Source: CAD feature listing. Evaluate the final solid. Frame: model axes, mm. A direction names the side the tool comes from. Coordinates: 2 decimals unless noted, no trailing zeros. Loops run counter-clockwise (first coordinate to the right, second up) from the corner with the lowest first, then second, coordinate; pieces in that order, holes last.
Autodesk Inventor part; units mm, degrees
ref_plane "YZ Plane" through (0, 0, 0) normal (1, 0, 0) x (0, 1, 0)
ref_plane "XZ Plane" through (0, 0, 0) normal (0, 1, 0) x (-1, 0, 0)
ref_plane "XY Plane" through (0, 0, 0) normal (0, 0, 1) x (1, 0, 0)
sketch "Boceto1" plane through (0, 0, 0) normal (0, 1, 0) x (-1, 0, 0)
  line L0 (-25, 24.85) -> (25, 24.85)
  line L1 (25, 24.85) -> (25, -24.85)
  line L2 (25, -24.85) -> (-25, -24.85)
  line L3 (-25, -24.85) -> (-25, 24.85)
  line L4 (-25, 24.85) -> (25, -24.85) construction
  line L5 (25, 24.85) -> (-25, -24.85) construction
  circle A0 centre (0, 0) radius 4.35
  dimension "d0" = 50
  dimension "d1" = 8.7
  dimension "d2" = 49.7
extrude "Extrusión1" add sketch "Boceto1" along normal blind 10
sketch "Boceto4" plane through (0, 0, 0) normal (0, -1, 0) x (1, 0, 0)
  line L0 (25, 24.85) -> (25, -24.85)
  line L1 (-25, -24.85) -> (-25, 24.85)
  line L2 (25, 24.85) -> (-25, 24.85)
  line L3 (-25, 24.85) -> (-25, 17.85)
  line L4 (-25, 17.85) -> (25, 17.85)
  line L5 (25, 17.85) -> (25, 24.85)
  line L6 (25, -24.85) -> (-25, -24.85)
  line L7 (25, -24.85) -> (-25, -24.85)
  line L8 (-25, -24.85) -> (-25, -17.85)
  line L9 (-25, -17.85) -> (25, -17.85)
  line L10 (25, -17.85) -> (25, -24.85)
  line L11 (25, -24.85) -> (-25, -24.85)
  line L12 (25, 24.85) -> (25, -24.85)
  line L13 (-25, 24.85) -> (25, 24.85)
  line L14 (-25, -24.85) -> (-25, 24.85)
  circle A0 centre (0, 0) radius 4.35
  point P0 (-25, -17.85)
  point P1 (25, -17.85)
  point P2 (-25, 24.85)
  dimension "d14" = 7
  dimension "d15" = 7
extrude "Extrusión4" [suppressed]
sketch "Boceto5" plane through (0, 0, 0) normal (0, 0, 1) x (1, 0, 0)
  circle A0 centre (18, -5.5) radius 2.7
  circle A1 centre (-18, -5.5) radius 2.7
  line L0 (20, -12) -> (-20, -12)
  line L1 (25, 0) -> (25, 10)
  line L2 (-25, 0) -> (-25, 10)
  point P0 (0, 0)
  point P1 (-25, 10)
  dimension "d19" = 6.5
  dimension "d20" = 5.4
  dimension "d21" = 7
  dimension "d22" = 7
extrude "Extrusión5" [suppressed]
sketch "Boceto6" plane through (0, 0, 0) normal (0, 0, 1) x (1, 0, 0)
  circle A0 centre (13, -5.5) radius 2.7
  circle A1 centre (13, -5.5) radius 4.65
  circle A2 centre (-13, -5.5) radius 2.7
  circle A3 centre (-13, -5.5) radius 4.65
  point P0 (0, 0)
  dimension "d25" = 9.3
extrude "Extrusión6" [suppressed]
fillet "Empalme2" [suppressed]
fillet "Empalme3" [suppressed]
sketch "Boceto8" plane through (0, 0, 0) normal (0, -1, 0) x (1, 0, 0)
  circle A0 centre (0, 0) radius 4.35
  line L0 (-25, -24.85) -> (-25, 24.85)
  line L1 (25, 24.85) -> (25, -24.85)
  circle A1 centre (0, 0) radius 7.5
  line L2 (25, -24.85) -> (-25, -24.85)
  line L3 (-25, 24.85) -> (25, 24.85)
  dimension "d30" = 15
extrude "Extrusión7" [suppressed]
fillet "Empalme4" [suppressed]
sketch "Boceto9" plane through (0, 10, 0) normal (0, 1, 0) x (1, 0, 0)
  circle A0 centre (0, 0) radius 8.125
  dimension "d34" = 16.25
extrude "Extrusión8" cut sketch "Boceto9" against normal blind 5
sketch "Boceto10" plane through (0, 0, 0) normal (0, -1, 0) x (1, 0, 0)
  circle A0 centre (-18.9971, -19.0029) radius 2.7
  circle A1 centre (-19.0029, 18.9971) radius 2.7
  circle A2 centre (19.0029, -18.9971) radius 2.7
  circle A3 centre (18.9971, 19.0029) radius 2.7
  point P0 (0, 0)
extrude "Extrusión9" cut sketch "Boceto10" against normal through all
fillet "Empalme5" radius 5 4 edges at (-25, 5, 24.85) (25, 5, 24.85) (25, 5, -24.85) (-25, 5, -24.85)
sketch "Boceto11" plane through (0, 0, 0) normal (0, -1, 0) x (1, 0, 0)
  circle A0 centre (19.0029, -18.9971) radius 2.7
  circle A1 centre (19.0029, -18.9971) radius 4.05
  line L0 (14.9529, -21.3354) -> (14.9529, -16.6588)
  line L1 (14.9529, -16.6588) -> (19.0029, -14.3206)
  line L2 (19.0029, -14.3206) -> (23.0529, -16.6588)
  line L3 (23.0529, -16.6588) -> (23.0529, -21.3354)
  line L4 (23.0529, -21.3354) -> (19.0029, -23.6737)
  line L5 (19.0029, -23.6737) -> (14.9529, -21.3354)
  point P0 (0, 0)
  dimension "d40" = 8.1
extrude "Extrusión10" cut sketch "Boceto11" against normal blind 4 contours A0 | A1 | L3 L4 A1 | A1 L2 L3 | A1 L1 L2 | L4 L5 A1 | A1 L0 L1 | L5 L0 A1
pattern_circular "Patrón circular1" count 4 over 360 about axis through (0, 0, 0) along (0, 1, 0) of "Extrusión10"
properties part number "Shoulderbottom"
Q1. Access query for faces 1 (the cylindrical face through (18.418, 6.958, -21.633)), 2 (the flat face through (-15.506, 1.972, -16.95)). Directions: +Z, -Z, +X, -X, +Y, -Y. A direction counts if a zero-diameter tool reaches every point of the face in a straight line with its end or side. Return the directions, or none.
Q2. Contact query for flat-ended pins moving along their axis: pin 1 Ø7 at (x, z) = (-19, 19) entering from +Y; pin 2 Ø8 at (x, z) = (2, -2.5) entering from +Y; pin 3 Ø4 at (x, z) = (-19, -17.5) entering from -Y. Output: stop coordinate, or through.
Q3. Section D-D, the plane z = -20.5. Return the cut outline in (x, y).
Q4. Section A-A, the plane y = 1.25. Count the separate pieces of the cut face and the enclosed holes in it, plus the area to 3 significant figures.
Q5. Section B-B, the plane z = 0. Return the cut outline in (x, y) (3 decimals), plus the area to 3 significant figures.
Q6. Draft query along Z for faces 3 (the flat face through (6, 10, 6)), 4 (the cylindrical face through (7.75, 7.54, -2.44)), 5 (the flat face through (0, 5, -24.85)). Return one class per face: +Z half, -Z half, draft (parallel to the pull), parting line (faces both ways), or undercut.
Q7. Section C-C, the plane x = 0. Return the cut outline in (y, z) (3 decimals).
Q8. Line query: line 1 along X through (y, z) = (7, 19); line 2 along X through (y, z) = (1.05, 0); line 3 along Z through (x, y) = (21, 1.25). Output: solid intervals per line, ascending.
Derived:
1. face 1: +Y, -Y
1. face 2: -Y
2. pin 1: stops at y = 10
2. pin 2: stops at y = 5
2. pin 3: stops at y = 4
3. outline: (-24.96, 0) - (-22.81, 0) - (-22.81, 4) - (-21.24, 4) - (-21.24, 10) - (-24.96, 10) - close; (-16.75, 4) - (-15.18, 4) - (-15.18, 0) - (14.95, 0) - (14.95, 4) - (16.76, 4) - (16.76, 10) - (-16.75, 10) - close; (21.25, 4) - (23.05, 4) - (23.05, 0) - (24.96, 0) - (24.96, 10) - (21.25, 10) - close
4. separate pieces: 1
4. enclosed holes: 5
4. area: 2,180 mm2
5. outline: (-25, 0) - (-4.35, 0) - (-4.35, 5) - (-8.125, 5) - (-8.125, 10) - (-25, 10) - close; (4.35, 0) - (25, 0) - (25, 10) - (8.125, 10) - (8.125, 5) - (4.35, 5) - close
5. area: 375 mm2
6. face 3: draft
6. face 4: undercut
6. face 5: -Z half
7. outline: (0, -24.85) - (10, -24.85) - (10, -8.125) - (5, -8.125) - (5, -4.35) - (0, -4.35) - close; (0, 4.35) - (5, 4.35) - (5, 8.125) - (10, 8.125) - (10, 24.85) - (0, 24.85) - close
8. line 1: x = -25 to -21.7, -16.3 to 16.3, 21.7 to 25
8. line 2: x = -25 to -4.35, 4.35 to 25
8. line 3: z = -24.75 to -22.52, -15.47 to 14.95, 23.05 to 24.75
